```python
from build123d import *

# Parameters (mm, degrees)
BOSS_EXTRUDE1_DEPTH             = 12.7
BOSS_EXTRUDE2_REACH             = 70.956
BOSS_EXTRUDE2_DIRECTION_2_REACH = 70.956
SKETCH5_W                       = 27.5
SKETCH5_H                       = 3
CUT_EXTRUDE1_DEPTH              = 6
FILLET2_R                       = 6.35
FILLET3_START                   = -16.25
FILLET3_DEPTH                   = 32.5
FILLET3_START_2                 = -29
FILLET3_2_DEPTH                 = 7.65
BOSS_EXTRUDE3_DEPTH             = 38.1
BOSS_EXTRUDE3_DEPTH_BACK        = 50.8
CUT_EXTRUDE2_REACH              = 96.662
SKETCH7_W                       = 20
SKETCH7_H                       = 31.75
FILLET4_R                       = 12.7
BOSS_EXTRUDE4_DEPTH             = 30
FILLET6_R                       = 6.35


with BuildPart() as part:
    # Sketch2 → Boss-Extrude1 (new, symmetric)
    with BuildSketch(Plane.XY):
        Polygon((-11.25, 7.44), (-11.25, -15), (11.25, -15), (11.25, 7.44), (16.25, 7.44), (16.25, -65.8), (-16.25, -65.8), (-16.25, 7.44), align=None)
    extrude(amount=BOSS_EXTRUDE1_DEPTH, both=True)

    # Boss-Extrude2: up to this face of the body (flat: up to its plane)
    boss_extrude2_end = Plane(part.part.faces().sort_by_distance((11.25, -3.78, 0))[0])
    # Sketch4 → Boss-Extrude2 (add, up to the picked face)
    with BuildSketch(Plane(origin=(0, 0, 0), x_dir=(0, 0, -1), z_dir=(1, 0, 0)), mode=Mode.PRIVATE) as boss_extrude2_sk1:
        Polygon((12.7, -15), (44.525, -15), (44.525, -4.262817999), (50.875, -4.262817999), (50.875, -21.35), (12.7, -21.35), align=None)
    boss_extrude2_tool1 = split(extrude(boss_extrude2_sk1.sketch, amount=BOSS_EXTRUDE2_REACH, mode=Mode.PRIVATE), bisect_by=boss_extrude2_end, keep=Keep.BOTH, mode=Mode.PRIVATE)
    add(boss_extrude2_tool1.solids().sort_by(Axis((0, -16.299514, -35.280605), (1, 0, 0)))[0])

    # Boss-Extrude2 direction 2: up to this face of the body (flat: up to its plane)
    boss_extrude2_direction_2_end = Plane(part.part.faces().sort_by_distance((-16.25, -29.18, 0))[0])
    # Sketch4 → Boss-Extrude2 direction 2 (add, up to the picked face)
    with BuildSketch(Plane(origin=(0, 0, 0), x_dir=(0, 0, -1), z_dir=(1, 0, 0)), mode=Mode.PRIVATE) as boss_extrude2_direction_2_sk1:
        Polygon((12.7, -15), (44.525, -15), (44.525, -4.262817999), (50.875, -4.262817999), (50.875, -21.35), (12.7, -21.35), align=None)
    boss_extrude2_direction_2_tool1 = split(extrude(boss_extrude2_direction_2_sk1.sketch, amount=-BOSS_EXTRUDE2_DIRECTION_2_REACH, mode=Mode.PRIVATE), bisect_by=boss_extrude2_direction_2_end, keep=Keep.BOTH, mode=Mode.PRIVATE)
    add(boss_extrude2_direction_2_tool1.solids().sort_by(Axis((0, -16.299514, -35.280605), (-1, 0, 0)))[0])

    # Sketch5 → Cut-Extrude1 (cut)
    with BuildSketch(Plane(origin=(0, -4.262817999, 0), x_dir=(1, 0, 0), z_dir=(0, 1, 0))):
        with Locations((-2.5, 47.7)):
            Rectangle(SKETCH5_W, SKETCH5_H)
    extrude(amount=-CUT_EXTRUDE1_DEPTH, mode=Mode.SUBTRACT)

    # Fillet2
    # the kernel refuses this fillet: 6.35 mm, written as the material it adds along each edge
    with BuildSketch(Plane(origin=(11.25, -15, -12.7), x_dir=(0, 0, -1), z_dir=(0, -1, 0))) as fillet2_piece_1:
        with BuildLine():
            CenterArc((6.204836823, 6.35), FILLET2_R, 192.274670215, 77.725329785)
            Line((0, 5), (0, 0))
            Line((0, 0), (6.204836823, 0))
        make_face()
    extrude(amount=6.35)

    # Fillet3: read off the stored shape, not the designer's step
    # Fillet3 outline → Fillet3 (add)
    with BuildSketch(Plane.YZ.offset(FILLET3_START)):
        with BuildLine():
            Line((-21.35, -12.7), (-27.7, -12.7))
            ThreePointArc((-27.7, -12.7), (-23.209871939, -14.559871939), (-21.35, -19.05))
            Line((-21.35, -19.05), (-21.35, -12.7))
        make_face()
    extrude(amount=FILLET3_DEPTH)

    # Fillet3 2 outline → Fillet3 2 (cut)
    with BuildSketch(Plane(origin=(0, 0, 0), x_dir=(1, 0, 0), z_dir=(0, 1, 0)).offset(FILLET3_START_2)):
        with BuildLine():
            Line((11.25, 21), (11.25, 18.904836823))
            ThreePointArc((11.25, 18.904836823), (12.655571335, 14.920476752), (16.250039425, 12.699991422))
            Line((16.250039425, 12.699991422), (18, 12.319260294))
            Line((18, 12.319260294), (18, 21))
            Line((18, 21), (11.25, 21))
        make_face()
    extrude(amount=FILLET3_2_DEPTH, mode=Mode.SUBTRACT)

    # Sketch6 → Boss-Extrude3 (add, two sides: drawn at the far end of the back side and taken through both)
    with BuildSketch(Plane.XY.offset(12.7).offset(-BOSS_EXTRUDE3_DEPTH_BACK)):
        Polygon((16.25, -65.8), (52.572, -65.8), (52.572, -4.05), (46.222, -4.05), (46.222, -35.8), (35.3, -35.8), (35.3, -4.05), (28.95, -4.05), (28.95, -35.8), (16.25, -35.8), align=None)
    extrude(amount=BOSS_EXTRUDE3_DEPTH + BOSS_EXTRUDE3_DEPTH_BACK)

    # Sketch7 → Cut-Extrude2 (cut, up to next)
    with BuildSketch(Plane.ZY.offset(-28.95), mode=Mode.PRIVATE) as cut_extrude2_sk1:
        with Locations((-28.1, -19.925)):
            Rectangle(SKETCH7_W, SKETCH7_H)
    cut_extrude2_tool1 = extrude(cut_extrude2_sk1.sketch, amount=-CUT_EXTRUDE2_REACH, mode=Mode.PRIVATE) & part.part
    add(cut_extrude2_tool1.solids().sort_by_distance((28.95, -19.925, -28.1))[0], mode=Mode.SUBTRACT)

    # Fillet4
    fillet4_edges = [part.edges().sort_by_distance(p)[0] for p in [
        (16.25, -50.8, -12.7),
    ]]
    fillet(fillet4_edges, radius=FILLET4_R)

    # Sketch8 → Boss-Extrude4 (add)
    with BuildSketch(Plane.XZ.offset(65.8)):
        Polygon((-16.25, 12.7), (16.25, 50.8), (16.25, 12.7), align=None)
    extrude(amount=-BOSS_EXTRUDE4_DEPTH)

    # Fillet6
    fillet6_edges = [part.edges().sort_by_distance(p)[0] for p in [
        (0, -35.8, 12.7),
    ]]
    fillet(fillet6_edges, radius=FILLET6_R)


solid = part.part
```
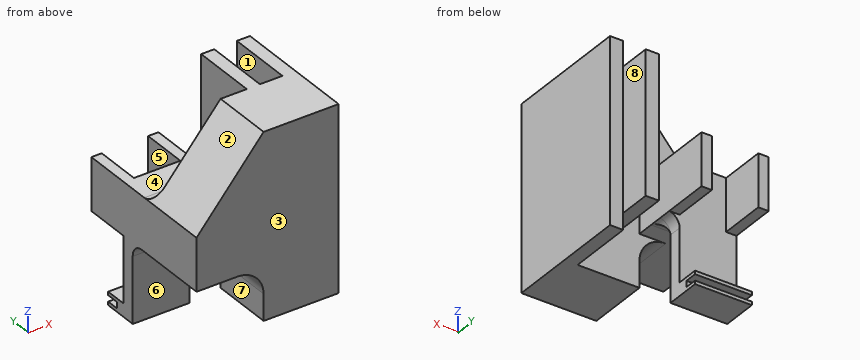
The model under review builds one solid part; all positions refer to its coordinate system, in mm. Face numbers are marked on the shaded views. A direction names the side the tool comes from. Round coordinates to 2 decimals unless told otherwise and drop trailing zeros. Order: outer loops, then holes, each group sorted by start corner. A loop starts at its lowest first (then second) coordinate and runs counter-clockwise, first axis right, second up. Notation, with made-up numbers: (85, 68.5) -> (113, 68.5) arc R17 cw to (113, 99.5) -> close; hole circle Ø3 at (43, 13). An arc over 180 degrees is marked (long way). Use a Markdown table: item, result.
Q1. For line 1 (X direction, y = -27.5, z = 9); line 2 (X direction, y = -7, z = -12); line 3 (Z direction, x = 8, y = -9) (3 decimals), list the stretches that pass through material, from the lowest coordinate up.
Values:
| item | result |
|---|---|
| line 1 | x = -16.25 to 16.25, 28.95 to 35.3, 46.22 to 52.57 |
| line 2 | x = -16.25 to -11.25, 11.25 to 16.25, 28.95 to 35.3, 46.22 to 52.57 |
| line 3 | z = -50.875 to -49.2, -46.2 to -44.525 |
Q2. Mouldability with a two-part tool opening along X and no side actions: class the marked faces 1, 2 and 3 as +X half, -X half, draft (parallel to the pull), parting line (faces both ways), or undercut.
Values:
| item | result |
|---|---|
| face 1 | undercut |
| face 2 | -X half |
| face 3 | draft |
Q3. Tool access review of the marked faces 4, 5, 6, 7 and 8: name each direction out of +Z, -Z, +X, -X, +Y, -Y from which nothing blocks a thin tool from reaching the whole face with its end or side.
Values:
| item | result |
|---|---|
| face 4 | +Z, -X, +Y |
| face 5 | +Z, +Y |
| face 6 | -Z, -X, -Y |
| face 7 | -Z, -X, +Y, -Y |
| face 8 | +Z, -Z, +Y |
Q4. We need section C-C on y = -6. Write out the cut boundary in (x, z) (3 decimals).
Values:
| item | result |
|---|---|
| outline | (-16.25, -50.875) -> (11.25, -50.875) -> (11.25, -49.2) -> (-16.25, -49.2) -> close; (-16.25, -46.2) -> (11.25, -46.2) -> (11.25, -44.525) -> (-16.25, -44.525) -> close; (-16.25, -12.7) -> (-11.25, -12.7) -> (-11.25, 12.7) -> (-16.25, 12.7) -> close; (11.25, -12.7) -> (16.25, -12.7) -> (16.25, 12.7) -> (11.25, 12.7) -> close; (28.95, -18.1) -> (35.3, -18.1) -> (35.3, 50.8) -> (28.95, 50.8) -> close; (46.222, -38.1) -> (52.572, -38.1) -> (52.572, 50.8) -> (46.222, 50.8) -> close |
Q5. We need section D-D on y = -39.5. Write out the cut boundary in (x, z).
Values:
| item | result |
|---|---|
| outline | (-16.25, -12.7) -> (3.55, -12.7) arc R12.7 cw to (16.25, -25.4) -> (16.25, -38.1) -> (52.57, -38.1) -> (52.57, 50.8) -> (16.25, 50.8) -> (-16.25, 12.7) -> close |
Q6. We need section B-B on z = -21.5. Write out the cut boundary in (x, y), then the cut area to 3 significant figures.
Values:
| item | result |
|---|---|
| outline | (-16.25, -21.35) -> (11.25, -21.35) -> (11.25, -15) -> (-16.25, -15) -> close; (15.64, -65.8) -> (52.57, -65.8) -> (52.57, -4.05) -> (46.22, -4.05) -> (46.22, -35.8) -> (15.64, -35.8) -> close |
| area | 1,480 mm^2 |
Q7. We need section A-A on y = -16.5. Write out the cut boundary in (x, z) (3 decimals), then the cut area to 3 significant figures.
Values:
| item | result |
|---|---|
| outline | (-16.25, -50.875) -> (11.25, -50.875) -> (11.25, -18.905) arc R6.35 cw to (16.25, -12.7) -> (16.25, 12.7) -> (-16.25, 12.7) -> close; (28.95, -18.1) -> (35.3, -18.1) -> (35.3, 50.8) -> (28.95, 50.8) -> close; (46.222, -38.1) -> (52.572, -38.1) -> (52.572, 50.8) -> (46.222, 50.8) -> close |
| area | 2,890 mm^2 |
Q8. Clearance check with flat-ended pins moving along their axes: P1, Ø1.3, axis at x = -2, z = -45.5, coming from the +Y side; P2, Ø5, axis at x = 51, z = 19, coming from the +Y side; P3, Ø1, axis at x = 38.5, y = -33.5, coming from the +Z side; P4, Ø1, axis at y = -40, z = -15, coming from the -X side. State where each tip first meets the part, or that it passes through.
Values:
| item | result |
|---|---|
| P1 | stops at y = -4.26 |
| P2 | stops at y = -4.05 |
| P3 | passes through |
| P4 | stops at x = 10.07 |
